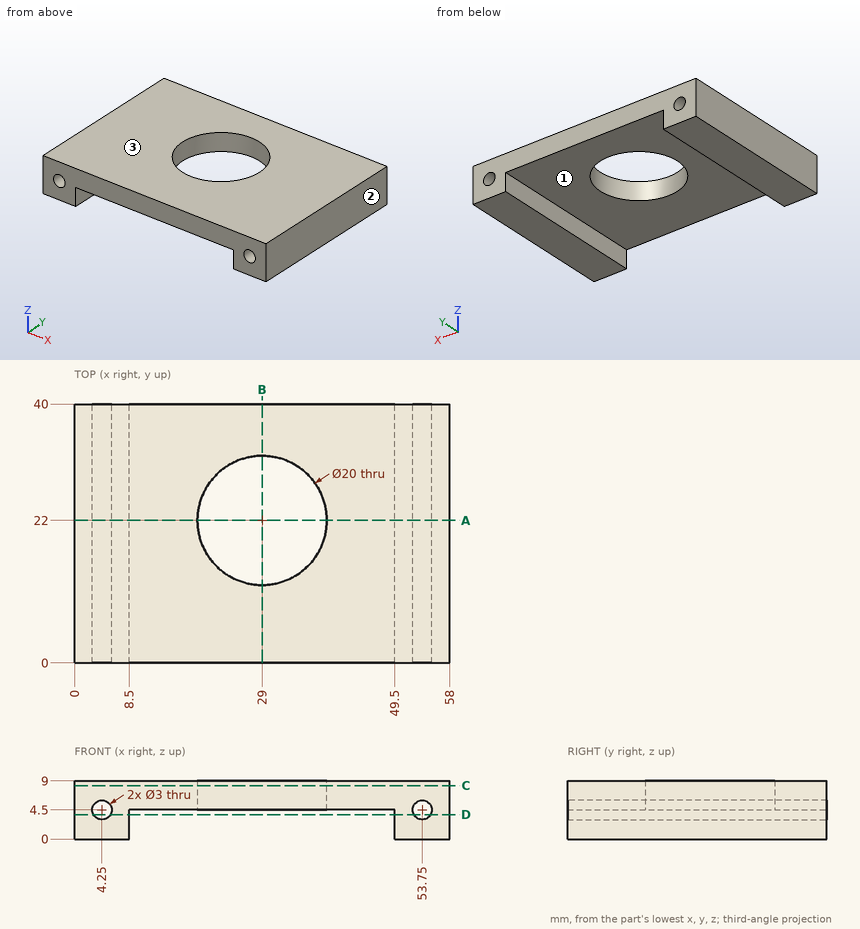
For this review, use the dimensioned drawing (mm, ordinates from the lowest corner) and the shaded views. Coordinates: 2 decimals unless noted, no trailing zeros. Order: outer loops, then holes, each group sorted by start corner. A loop starts at its lowest first (then second) coordinate and runs counter-clockwise, first axis right, second up. Notation, with made-up numbers: (57.25, 57) - (75.25, 57) arc R16 cw to (75.25, 70) - close; hole circle Ø7 at (82, 40.25). An arc over 180 degrees is marked (long way). Answer as a JSON object with one key per item and string values. Group by question number.
1. We need section D-D on z = 3.75. State the section outline as (x, y) points, then the cut area to 3 significant figures.
2. We need section A-A on y = 22. State the section outline as (x, z) points, then the cut area to 3 significant figures.
3. For probe 1 along Y at (x, z) = (29, 5.5); probe 2 along X at (y, z) = (34, 1.25); probe 3 along X at (y, z) = (21.5, 3.5), list the stretches that pass through material, from the lowest coordinate up.
4. We need section C-C on z = 8.25. State the section outline as (x, y) points, then the cut area to 3 significant figures.
5. Clearance check with flat-ended pins moving along their axes: P1, Ø12, axis at x = 17, y = 13.5, coming from the -Z side; P2, Ø1, axis at x = 23.5, z = 2.5, coming from the +Y side. State where each tip first meets the part, or that it passes through.
6. The part is to be moulded in two halves that separate along X. For the marked faces 1, 2 and 3, say which applies: pulls with the +X half, pulls with the -X half, needs draft (parallel to the pull), parting line crosses it, or undercut.
7. We need section B-B on x = 29. State the section outline as (y, z) points.
Final values:
{
 "1": {"outline": "(0, 0) - (2.95, 0) - (2.95, 40) - (0, 40) - close; (5.55, 0) - (8.5, 0) - (8.5, 40) - (5.55, 40) - close; (49.5, 0) - (52.45, 0) - (52.45, 40) - (49.5, 40) - close; (55.05, 0) - (58, 0) - (58, 40) - (55.05, 40) - close", "area": "472 mm²"},
 "2": {"outline": "(0, 0) - (8.5, 0) - (8.5, 4.5) - (19, 4.5) - (19, 9) - (0, 9) - close; (39, 4.5) - (49.5, 4.5) - (49.5, 0) - (58, 0) - (58, 9) - (39, 9) - close; hole circle Ø3 at (4.25, 4.5); hole circle Ø3 at (53.75, 4.5)", "area": "233 mm²"},
 "3": {"probe 1": "0 to 12, 32 to 40", "probe 2": "0 to 8.5, 49.5 to 58", "probe 3": "0 to 3.13, 5.37 to 8.5, 49.5 to 52.63, 54.87 to 58"},
 "4": {"outline": "(0, 0) - (58, 0) - (58, 40) - (0, 40) - close; hole circle Ø20 at (29, 22)", "area": "2,010 mm²"},
 "5": {"P1": "z = 4.5", "P2": "through"},
 "6": {"face 1": "undercut", "face 2": "pulls with the +X half", "face 3": "needs draft"},
 "7": {"outline": "(0, 4.5) - (12, 4.5) - (12, 9) - (0, 9) - close; (32, 4.5) - (40, 4.5) - (40, 9) - (32, 9) - close"}
}
